from build123d import *

# Parameters (mm, degrees)
F0_R     = 5.475
F1_DEPTH = 1.35
F2_R     = 2.75
F3_DEPTH = 6
F4_R     = 6.375
F5_DEPTH = 3.45
F6_R     = 3.73
F7_DEPTH = 69


with BuildPart() as f1:
    # F0 (on Top) → F1 (new body)
    with BuildSketch(Plane.XY):
        Circle(F0_R)
    extrude(amount=F1_DEPTH)

    # F2 (on Top) → F3 (join)
    with BuildSketch(Plane.XY):
        Circle(F2_R)
    extrude(amount=F3_DEPTH)

    # F4 (on face) → F5 (join)
    with BuildSketch(Plane.XY.offset(6)):
        Circle(F4_R)
    extrude(amount=F5_DEPTH)

    # F6 (on face) → F7 (join)
    with BuildSketch(Plane.XY.offset(9.45)):
        Circle(F6_R)
    extrude(amount=F7_DEPTH)


solid = f1.part
Input: part model. Units: mm. Frame: model coordinates. A direction names the side the tool comes from. Give positions to 0.01 mm unless a question says otherwise; leave off trailing zeros. Order: outer loops, then holes, each group sorted by start corner. A loop starts at its lowest first (then second) coordinate and runs counter-clockwise, first axis right, second up. Notation, with made-up numbers: (-31, 22) -> (-7, 22) arc R31 cw to (-7, 47) -> close; hole circle Ø2 at (-25, 70.25). An arc over 180 degrees is marked (long way). Use one line per item in the form item = value.
1) Reachability of faces 4 (the flat face through (3, -1, 6)), 5 (the flat face through (0, 0, 0)), 6 (the cylindrical face through (-4.345, -3.331, 0.666)), 7 (the cylindrical face through (-0.486, 3.698, 43.467)) from +Z, -Z, +X, -X, +Y, -Y: full face, straight path, thin tool, end or side. Return the list, or none.
Response values:
face_4 = none
face_5 = -Z, +X, -X, +Y, -Y
face_6 = -Z
face_7 = +Z
2) First-contact query: pin 1 Ø6 at (x, z) = (-2, 12.5) entering from -Y; pin 2 Ø1 at (x, z) = (2.5, 21.5) entering from +Y; pin 3 Ø3 at (x, z) = (-1.5, 50) entering from +Y. Flat tips, straight axial feed; report the tip coordinate or a pass-through.
Response values:
pin_1 = -3.73
pin_2 = 3.15
pin_3 = 3.73
3) Section C-C, the plane z = 37. Return loops of the section in (x, y).
Response values:
outline = circle Ø7.46 at (0, 0)
4) Mould query, pull axis Z, two halves, no side actions, for faces 1 (the flat face through (0, 0, 78.45)), 2 (the cylindrical face through (-0.596, -2.685, 3.642)), 3 (the cylindrical face through (-1.382, -6.223, 7.701)). Classes: pulls with the +Z half, pulls with the -Z half, needs draft (parallel to the pull), parting line crosses it, or undercut.
Response values:
face_1 = pulls with the +Z half
face_2 = undercut
face_3 = needs draft
5) Section A-A, the plane y = 0. Return loops of the section in (x, z) (3 decimals).
Response values:
outline = (-6.375, 6) -> (-2.75, 6) -> (-2.75, 1.35) -> (-5.475, 1.35) -> (-5.475, 0) -> (5.475, 0) -> (5.475, 1.35) -> (2.75, 1.35) -> (2.75, 6) -> (6.375, 6) -> (6.375, 9.45) -> (3.73, 9.45) -> (3.73, 78.45) -> (-3.73, 78.45) -> (-3.73, 9.45) -> (-6.375, 9.45) -> close
6) Line query: probe 1 along Z at (x, y) = (-5, 1); probe 2 along Y at (x, z) = (0, 74); probe 3 along X at (y, z) = (3.25, 9). Output: solid intervals per line, ascending.
Response values:
probe_1 = 0 to 1.35, 6 to 9.45
probe_2 = -3.73 to 3.73
probe_3 = -5.48 to 5.48
